Input: part model. Units: mm. Frame: model coordinates. A direction names the side the tool comes from. Coordinates: 2 decimals unless noted, no trailing zeros. Write each loop counter-clockwise with the first axis right and the second up, starting at its lowest first coordinate (ties: lowest second). Pieces come first, ordered by that corner, then holes. Notation, with made-up numbers: (88.5, -25.75) - (104.5, -25.75) arc R23 cw to (104.5, 2.25) - close; hole circle Ø5 at (80, 82.5). An arc over 180 degrees is marked (long way). Use a Markdown table: item, result. Add a question column.
Q1. Pin query (flat end, axial travel): P1, Ø3.5, axis at x = -124.72, y = 0, coming from the +Z side; P2, Ø2.5, axis at x = -110, z = 2, coming from the -Y side; P3, Ø4, axis at y = 22, z = 2.5, coming from the -X side; P4, Ø10, axis at x = -94, y = 15.5, coming from the +Z side. Return the tip coordinate at first contact, or that it passes through.
Q2. Section query A-A (y = 0). Give the number of separate pieces and of enclosed holes in the cut face, then the cut area to 3 significant figures.
Q3. Mould query, pull axis Y, two halves, no side actions, for faces 1 (the face through (-97.28, 2.73, 5.49)), 2 (the face through (-97, 0, 4.762)), 3 (the face through (-78.22, -8.09, 2.35)). Classes: released by +Y, released by -Y, zero draft, split by the parting line, or undercut.
Q4. Material intervals for probe 1 along Y at (x, z) = (-102.5, 10.5); probe 2 along Z at (x, y) = (-146.5, -2); probe 3 along Y at (x, z) = (-126, 1.75), sorted ascending. Write a range as from..to.
Q5. Section query D-D (x = -124.5). Return the cut outline in (y, z).
Q6. Section query B-B (x = -138.5). Return the cut outline in (y, z), then the cut area to 3 significant figures.
Q7. Set-up query: faces 4 (the face through (-68.24, 25.79, 2.35)), 5 (the face through (-97, -1.968, 9)), 6 (the face through (-82, 0, 4.762)). Return all of +Z, -Z, +X, -X, +Y, -Y with unobstructed straight access to the full face (end or side cutting, diameter ignored); none if empty.
from build123d import *

# Parameters (mm, degrees)
SKETCH1_R           = 1.905
BOSS_EXTRUDE1_DEPTH = 4.7625
BOSS_EXTRUDE2_DEPTH = 1.9685
FILLET1_R           = 2.54


with BuildPart() as part:
    # Sketch1 → Boss-Extrude1 (new body)
    with BuildSketch(Plane.XY):
        with BuildLine():
            Line((-71.045544716, 27.335394647), (-63.656604316, 27.335394647))
            ThreePointArc((-63.656604316, 27.335394647), (-60.962527479, 26.219471483), (-59.846604316, 23.525394647))
            Line((-59.846604316, 23.525394647), (-59.846604316, 0))
            Line((-59.846604316, 0), (-59.846604316, -23.525394647))
            ThreePointArc((-59.846604316, -23.525394647), (-60.962527479, -26.219471483), (-63.656604316, -27.335394647))
            Line((-63.656604316, -27.335394647), (-71.045544716, -27.335394647))
            ThreePointArc((-71.045544716, -27.335394647), (-73.499934786, -26.439510188), (-74.800072929, -24.173173852))
            add(Edge.make_bspline(
                [(-76.255398054, -12.219815998), (-75.950115276, -16.245345964), (-75.476568023, -20.252208344), (-74.800072929, -24.173173852)],
                knots=[0.13080804, 0.13080804, 0.13080804, 0.13080804, 0.259951787, 0.259951787, 0.259951787, 0.259951787], degree=3))
            ThreePointArc((-76.255398054, -12.219815998), (-78.270195904, -8.04319485), (-82.587216381, -6.35))
            Line((-82.587216381, -6.35), (-152.901202739, -6.35))
            ThreePointArc((-152.901202739, -6.35), (-159.251202739, 0), (-152.901202739, 6.35))
            Line((-152.901202739, 6.35), (-82.587216381, 6.35))
            ThreePointArc((-82.587216381, 6.35), (-78.270195904, 8.04319485), (-76.255398054, 12.219815998))
            add(Edge.make_bspline(
                [(-74.800072929, 24.173173852), (-75.476568023, 20.252208344), (-75.950115276, 16.245345964), (-76.255398054, 12.219815998)],
                knots=[0.740048213, 0.740048213, 0.740048213, 0.740048213, 0.86919196, 0.86919196, 0.86919196, 0.86919196], degree=3))
            ThreePointArc((-74.800072929, 24.173173852), (-73.499934786, 26.439510188), (-71.045544716, 27.335394647))
        make_face()
        with Locations((-152.901202739, 0)):
            Circle(SKETCH1_R, mode=Mode.SUBTRACT)
        with Locations((-138.811822739, 0)):
            Circle(SKETCH1_R, mode=Mode.SUBTRACT)
        with Locations((-124.722442739, 0)):
            Circle(SKETCH1_R, mode=Mode.SUBTRACT)
        with Locations((-110.633062739, 0)):
            Circle(SKETCH1_R, mode=Mode.SUBTRACT)
        with Locations((-96.543682739, 0)):
            Circle(SKETCH1_R, mode=Mode.SUBTRACT)
        with Locations((-82.454302739, 0)):
            Circle(SKETCH1_R, mode=Mode.SUBTRACT)
        with BuildLine():
            Line((-69.905853527, -24.160394647), (-69.905853527, -17.810394647))
            ThreePointArc((-69.905853527, -17.810394647), (-68.273903527, -16.178444647), (-66.641953527, -17.810394647))
            Line((-66.641953527, -17.810394647), (-66.641953527, -24.160394647))
            ThreePointArc((-66.641953527, -24.160394647), (-68.273903527, -25.792344647), (-69.905853527, -24.160394647))
        make_face(mode=Mode.SUBTRACT)
        with BuildLine():
            Line((-69.905853527, 24.160394647), (-69.905853527, 17.810394647))
            ThreePointArc((-69.905853527, 17.810394647), (-68.273903527, 16.178444647), (-66.641953527, 17.810394647))
            Line((-66.641953527, 17.810394647), (-66.641953527, 24.160394647))
            ThreePointArc((-66.641953527, 24.160394647), (-68.273903527, 25.792344647), (-69.905853527, 24.160394647))
        make_face(mode=Mode.SUBTRACT)
    extrude(amount=BOSS_EXTRUDE1_DEPTH)

    # Sketch2 → Boss-Extrude2 (add, symmetric)
    with BuildSketch(Plane(origin=(0, 0, 0), x_dir=(1, 0, 0), z_dir=(0, 1, 0))):
        with BuildLine():
            Line((-66.196604316, -4.7625), (-127.501202739, -4.7625))
            ThreePointArc((-127.501202739, -4.7625), (-96.848903527, -11.199497248), (-66.196604316, -4.7625))
        make_face()
    extrude(amount=BOSS_EXTRUDE2_DEPTH, both=True)

    # Fillet1
    fillet1_edges = [part.edges().sort_by_distance(p)[0] for p in [
        (-96.848903527, -1.9685, 4.7625),
        (-96.848903527, 1.9685, 4.7625),
    ]]
    fillet(fillet1_edges, radius=FILLET1_R)


solid = part.part
Values follow:
| question | item | result |
|---|---|---|
| 1 | P1 | z = 6.58 |
| 1 | P2 | y = -6.35 |
| 1 | P3 | x = -75.44 |
| 1 | P4 | through |
| 2 | separate pieces | 3 |
| 2 | enclosed holes | 0 |
| 2 | area | 630 mm2 |
| 3 | face 1 | released by +Y |
| 3 | face 2 | undercut |
| 3 | face 3 | released by -Y |
| 4 | probe 1 | -1.97..1.97 |
| 4 | probe 2 | 0..4.76 |
| 4 | probe 3 | -6.35..-1.41, 1.41..6.35 |
| 5 | outline | (-6.35, 0) - (-1.89, 0) - (-1.89, 4.76) - (1.89, 4.76) - (1.89, 0) - (6.35, 0) - (6.35, 4.76) - (4.51, 4.76) arc R2.54 cw to (2.32, 6.01) - (-2.32, 6.01) arc R2.54 cw to (-4.51, 4.76) - (-6.35, 4.76) - close |
| 6 | outline | (-6.35, 0) - (-1.88, 0) - (-1.88, 4.76) - (-6.35, 4.76) - close; (1.88, 0) - (6.35, 0) - (6.35, 4.76) - (1.88, 4.76) - close |
| 6 | area | 42.6 mm2 |
| 7 | face 4 | +Z, -Z |
| 7 | face 5 | +Z, +X, -X, -Y |
| 7 | face 6 | -Z |
